```python
from build123d import *

# Parameters (mm, degrees)
SKETCH002_W  = 42
SKETCH002_H  = 24.6
PAD002_DEPTH = 7.4
FILLET004_R  = 8
SKETCH_W     = 50
SKETCH_H     = 50
PAD_DEPTH    = 5
FILLET_R     = 8
SKETCH001_W  = 42
SKETCH001_H  = 30
PAD001_DEPTH = 10
SKETCH003_W  = 40
SKETCH003_H  = 40
POCKET_DEPTH = 2
FILLET005_R  = 8
FILLET006_R  = 3
FILLET007_R  = 2
FILLET008_R  = 3


with BuildPart() as body001:
    # Sketch002 → Pad002 (new body)
    with BuildSketch(Plane.XY):
        with Locations((3, 0)):
            Rectangle(SKETCH002_W, SKETCH002_H)
    extrude(amount=PAD002_DEPTH)

    # Fillet004
    fillet004_edges = [body001.edges().sort_by_distance(p)[0] for p in [
        (-18, 12.3, 3.7),
        (-18, -12.3, 3.7),
    ]]
    fillet(fillet004_edges, radius=FILLET004_R)


with BuildPart() as body001_1:
    # Body001 placement: moved
    add(body001.part.moved(Location((0, 0, 5))))


with BuildPart() as body:
    # Sketch → Pad (new body)
    with BuildSketch(Plane.XY):
        Rectangle(SKETCH_W, SKETCH_H)
    extrude(amount=PAD_DEPTH)

    # Fillet
    fillet_edges = [body.edges().sort_by_distance(p)[0] for p in [
        (25, 25, 2.5),
        (25, -25, 2.5),
        (-25, 25, 2.5),
        (-25, -25, 2.5),
    ]]
    fillet(fillet_edges, radius=FILLET_R)

    # Sketch001 (on Face5 of Fillet) → Pad001 (join)
    with BuildSketch(Plane.XY.offset(5)):
        with Locations((-1, 0)):
            Rectangle(SKETCH001_W, SKETCH001_H)
    extrude(amount=PAD001_DEPTH)

    # Sketch003 → Pocket (cut)
    with BuildSketch(Plane(origin=(0, 0, 0), x_dir=(1, 0, 0), z_dir=(0, 0, -1))):
        Rectangle(SKETCH003_W, SKETCH003_H)
    extrude(amount=-POCKET_DEPTH, mode=Mode.SUBTRACT)

    # Boolean: cut Body001
    add(body001_1.part, mode=Mode.SUBTRACT)

    # Fillet005
    fillet005_edges = [body.edges().sort_by_distance(p)[0] for p in [
        (-22, 15, 10),
        (-22, -15, 10),
    ]]
    fillet(fillet005_edges, radius=FILLET005_R)

    # Fillet006
    fillet006_edges = [body.edges().sort_by_distance(p)[0] for p in [
        (-20, -20, 1),
        (-20, 20, 1),
        (20, 20, 1),
        (20, -20, 1),
    ]]
    fillet(fillet006_edges, radius=FILLET006_R)

    # Fillet007
    fillet007_edges = [body.edges().sort_by_distance(p)[0] for p in [
        (0, -25, 5),
    ]]
    fillet(fillet007_edges, radius=FILLET007_R)

    # Fillet008
    fillet008_edges = [body.edges().sort_by_distance(p)[0] for p in [
        (3, -15, 15),
    ]]
    fillet(fillet008_edges, radius=FILLET008_R)


solid = body.part
```
Source: CAD feature listing. Evaluate the final solid. Frame: model axes, mm. A direction names the side the tool comes from. Give positions to 0.01 mm unless a question says otherwise; leave off trailing zeros. Write each loop counter-clockwise with the first axis right and the second up, starting at its lowest first coordinate (ties: lowest second). Pieces come first, ordered by that corner, then holes. Notation, with made-up numbers: (-39.5, 74) - (-0.5, 74) arc R17 cw to (-0.5, 89) - close; hole circle Ø4 at (-19, 67.5). An arc over 180 degrees is marked (long way). One line per item, written item: value. Start each with the question number.
Q1. Section query C-C, the plane y = -1. Return the cut outline in (x, z).
Q2. Set-up query: faces 4 (the face through (22.594, -22.719, 1.521)), 5 (the face through (-15.719, 9.894, 8.752)), 6 (the face through (-19.594, 12.719, 8.549)), 7 (the face through (-22.719, 22.594, 1.521)), 8 (the face through (3, -15, 8)). Return all of +Z, -Z, +X, -X, +Y, -Y with unobstructed straight access to the full face (end or side cutting, diameter ignored); none if empty.
Q3. Section query B-B, the plane z = 9.75. Return the cut outline in (x, y), then the cut area to 3 significant figures.
Q4. Section query D-D, the plane x = -12. Return the cut outline in (y, z).
Q5. Material intervals for probe 1 along Z at (x, y) = (12, 9.5); probe 2 along Y at (x, z) = (-6, 5.25); probe 3 along Z at (x, y) = (-1, 21), sorted ascending. Write a range as from..to.
Q6. Draft query along Y for faces 1 (the face through (-19.594, -12.719, 8.549)), 2 (the face through (22.719, 22.594, 1.521)), 3 (the face through (0, 0, 5)). Return one class per face: +Y half, -Y half, draft (parallel to the pull), parting line (faces both ways), or undercut.
Q7. Section query A-A, the plane x = 14.5. Return the cut outline in (y, z).
Q8. First-contact query: pin 1 Ø3.5 at (x, z) = (-5, 8.5) entering from -Y; pin 2 Ø12.5 at (x, y) = (-0.5, -1.5) entering from -Z; pin 3 Ø5.5 at (y, z) = (-1, 8) entering from -X. Flat tips, straight axial feed; report the tip coordinate or a pass-through.
Answer:
1. outline: (-25, 0) - (-20, 0) - (-20, 2) - (20, 2) - (20, 0) - (25, 0) - (25, 3) arc R2 ccw to (23, 5) - (-18, 5) - (-18, 12.4) - (20, 12.4) - (20, 15) - (-19, 15) arc R3 ccw to (-22, 12) - (-22, 5) - (-23, 5) arc R2 ccw to (-25, 3) - close
2. face 4: +Z, -Z, +X, -Y
2. face 5: +X
2. face 6: +Z, -X, +Y
2. face 7: +Z, -Z, -X, +Y
2. face 8: +Z, +X, -X, -Y
3. outline: (-22, -7) arc R8 ccw to (-14, -15) - (20, -15) - (20, -12.3) - (-10, -12.3) arc R8 cw to (-18, -4.3) - (-18, 4.3) arc R8 cw to (-10, 12.3) - (20, 12.3) - (20, 15) - (-14, 15) arc R8 ccw to (-22, 7) - close
3. area: 325 mm2
4. outline: (-25, 0) - (-20, 0) - (-20, 2) - (20, 2) - (20, 0) - (25, 0) - (25, 3) arc R2 ccw to (23, 5) - (15, 5) - (15, 12) arc R3 ccw to (12, 15) - (-12, 15) arc R3 ccw to (-15, 12) - (-15, 5) - (-23, 5) arc R2 ccw to (-25, 3) - close; hole (-12.05, 5) - (12.05, 5) - (12.05, 12.4) - (-12.05, 12.4) - close
5. probe 1: z = 2..5, 12.4..15
5. probe 2: y = -15..-12.3, 12.3..15
5. probe 3: z = 0..5
6. face 1: -Y half
6. face 2: +Y half
6. face 3: undercut
7. outline: (-25, 0) - (-20, 0) - (-20, 2) - (20, 2) - (20, 0) - (25, 0) - (25, 3) arc R2 ccw to (23, 5) - (15, 5) - (15, 12) arc R3 ccw to (12, 15) - (-12, 15) arc R3 ccw to (-15, 12) - (-15, 5) - (-23, 5) arc R2 ccw to (-25, 3) - close; hole (-12.3, 5) - (12.3, 5) - (12.3, 12.4) - (-12.3, 12.4) - close
8. pin 1: stops at y = -15
8. pin 2: stops at z = 2
8. pin 3: stops at x = -22
